Source: CAD feature listing. Evaluate the final solid. Frame: model axes, mm. Give positions to 0.01 mm unless a question says otherwise; leave off trailing zeros. Loops run counter-clockwise (first coordinate to the right, second up) from the corner with the lowest first, then second, coordinate; pieces in that order, holes last. Notation, with made-up numbers: M 68,-4.75 L 84,-4.75 A15 cw 84,2.25 Z; hole C 73,-17 d9. An arc over 180 degrees is marked long. Answer in a Markdown table with one row per item.
Autodesk Inventor part; units mm, degrees
ref_plane "YZ Plane" through (0, 0, 0) normal (1, 0, 0) x (0, 1, 0)
ref_plane "XZ Plane" through (0, 0, 0) normal (0, 1, 0) x (-1, 0, 0)
ref_plane "XY Plane" through (0, 0, 0) normal (0, 0, 1) x (1, 0, 0)
sketch "Sketch1" plane through (0, 0, 0) normal (0, 0, 1) x (1, 0, 0)
  line L0 (0, 0) -> (-126.365, 0)
  line L1 (-126.365, 0) -> (-126.365, -25.4)
  line L2 (-126.365, -25.4) -> (0, -25.4)
  line L3 (0, -25.4) -> (0, 0)
  dimension "d0" = 126.365
  dimension "d1" = 25.4
extrude "Extrusion1" add sketch "Sketch1" along normal blind 3.175
sketch "Sketch2" plane through (0, 0, 0) normal (0, 0, -1) x (-1, 0, 0)
  circle A0 centre (38.1, -12.7) radius 3.3734
  circle A1 centre (12.7, -12.7) radius 3.3734
  line L0 (0, 0) -> (126.365, 0)
  line L1 (0, -25.4) -> (0, 0)
  dimension "d4" = 6.7469
  dimension "d5" = 12.7
  dimension "d6" = 12.7
  dimension "d7" = 25.4
  dimension "d8" = 12.7
extrude "Extrusion2" cut sketch "Sketch2" against normal blind 3.175
properties part number "supportbeam2" material "Aluminum 6061"
Q1. Contact query for a flat-ended pin moving along its axis: pin 1 Ø6 at (x, y) = (-38.1, -12.7) entering from +Z. Output: stop coordinate, or through.
Values follow:
| item | result |
|---|---|
| pin 1 | through |
Q2. Section query B-B (x = -12.7). Output: boundary loops of the cut face in (y, z) (3 decimals), plus the area to 3 significant figures.
Values follow:
| item | result |
|---|---|
| outline | M -25.4,0 L -16.073,0 L -16.073,3.175 L -25.4,3.175 Z; M -9.327,0 L 0,0 L 0,3.175 L -9.327,3.175 Z |
| area | 59.2 mm^2 |
Q3. Section query A-A (y = -12.7). Output: boundary loops of the cut face in (x, z) (3 decimals), plus the area to 3 significant figures.
Values follow:
| item | result |
|---|---|
| outline | M -126.365,0 L -41.473,0 L -41.473,3.175 L -126.365,3.175 Z; M -34.727,0 L -16.073,0 L -16.073,3.175 L -34.727,3.175 Z; M -9.327,0 L 0,0 L 0,3.175 L -9.327,3.175 Z |
| area | 358 mm^2 |
Q4. Mould query, pull axis X, two halves, no side actions, for faces 1 (the cylindrical face through (-12, -16, 2)), 2 (the flat face through (0, -13, 2)), 3 (the flat face through (-64, -13, 0)). Classes: +X half, -X half, draft (parallel to the pull), parting line (faces both ways), or undercut.
Values follow:
| item | result |
|---|---|
| face 1 | undercut |
| face 2 | +X half |
| face 3 | draft |
Q5. Ray query, probe 1 along Y at (x, z) = (-12.7, 1.35); probe 2 along X at (y, z) = (-10.5, 1.85) (3 decimals); probe 3 along X at (y, z) = (-11.75, 2.05) (3 decimals). Return the intervals inside material, ascending. Write a range as from..to.
Values follow:
| item | result |
|---|---|
| probe 1 | -25.4..-16.07, -9.33..0 |
| probe 2 | -126.365..-40.657, -35.543..-15.257, -10.143..0 |
| probe 3 | -126.365..-41.337, -34.863..-15.937, -9.463..0 |
